Can you work these out from the drawing? Everything is in mm from the part's minimum corner. Give positions to 0.01 mm unless a question says otherwise; leave off trailing zeros. Write each loop counter-clockwise with the first axis right and the second up, starting at its lowest first coordinate (ties: lowest second). Pieces come first, ordered by that corner, then holes. Notation, with made-up numbers: (86, 64.5) - (136, 64.5) arc R11 cw to (136, 78.5) - close; hole circle Ø4 at (52, 35.25). An arc over 180 degrees is marked (long way). Write each question's results on one line, items separated by ' | '. Start each with the question number.
Item 1: Suppose I cut it at A-A on z = 12.5. List the corners of the cut face in (x, y) for me, then the cut area to 3 significant figures.
Item 2: Will these pins go through, and if not, where does the flat tip stop? P1, Ø2, axis at y = 41, z = 12, coming from the -X side; P2, Ø2, axis at x = 11.5, y = 35, coming from the -Z side; P3, Ø5, axis at x = 24.5, z = 9.5, coming from the -Y side; P4, Ø1, axis at y = 34.5, z = 23, coming from the +X side.
Item 3: Please list where these lines run through material, in increasing order: line 1 along X through (y, z) = (29, 30); line 2 along Y through (x, z) = (33.5, 14); line 3 along X through (y, z) = (53.5, 17).
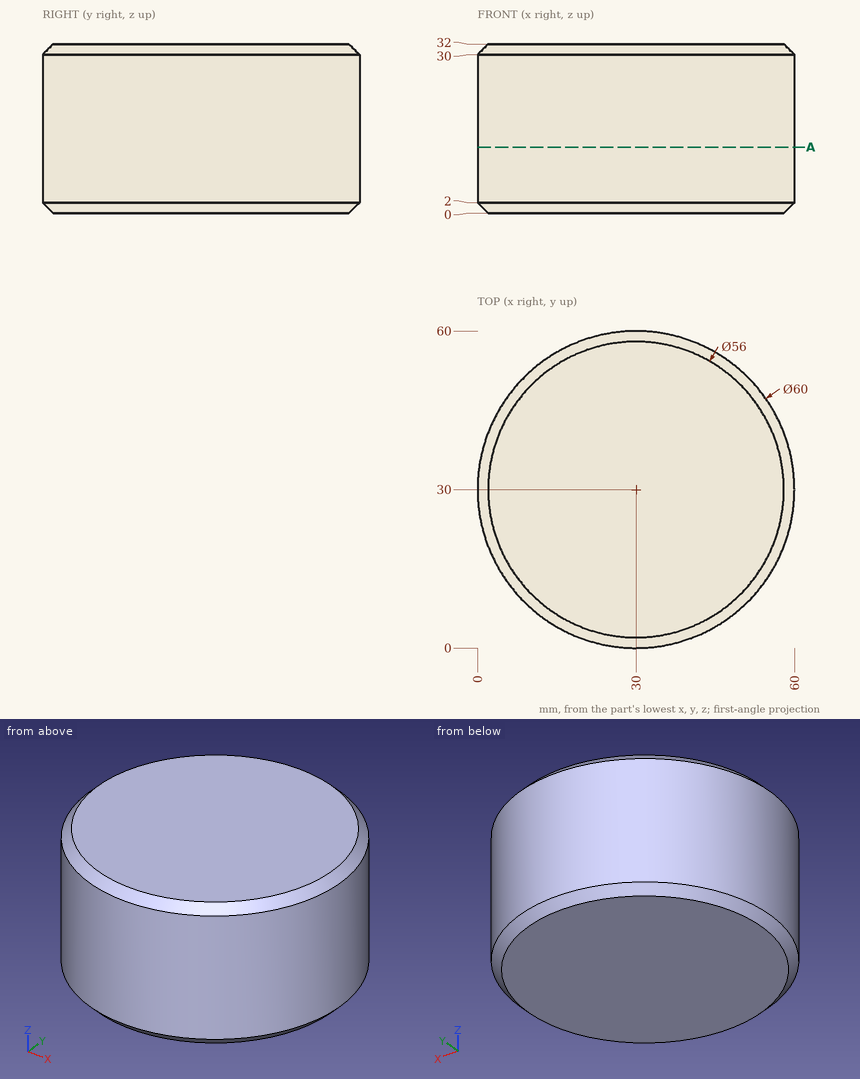
Checked values:
1) outline: circle Ø60 at (30, 30) | area: 2,830 mm^2
2) P1: stops at x = 1.72 | P2: stops at z = 0 | P3: stops at y = 0.15 | P4: stops at x = 59.73
3) line 1: x = 0.02 to 59.98 | line 2: y = 0.2 to 59.8 | line 3: x = 11.35 to 48.65
